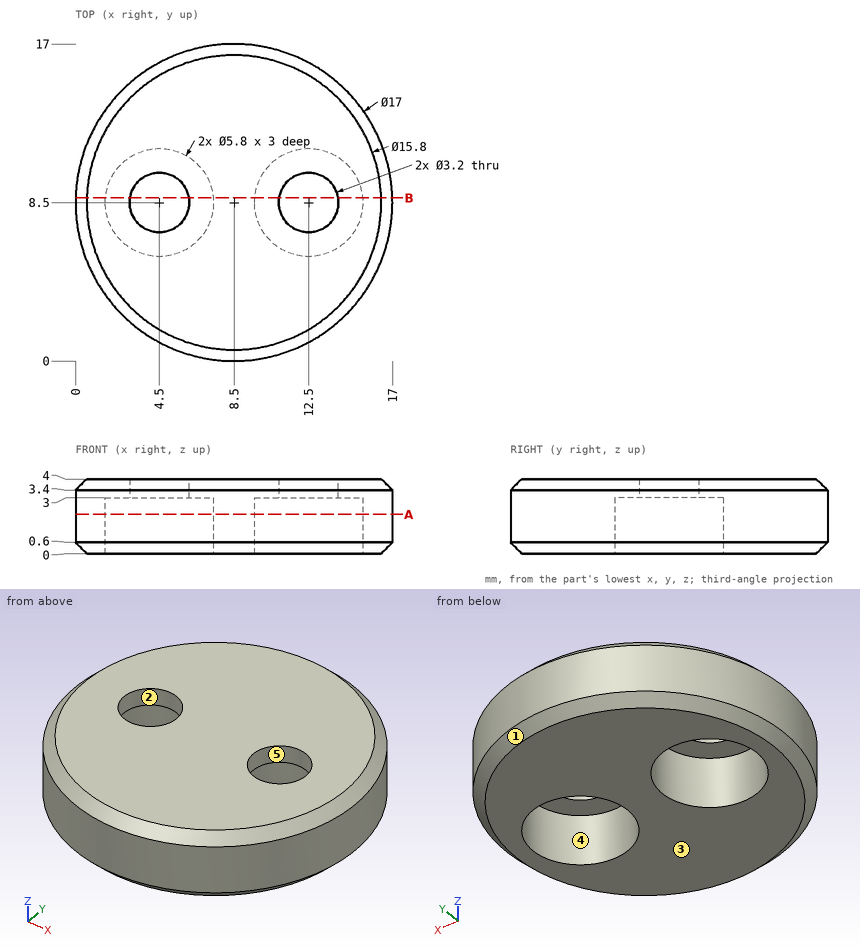
Geometry check sheet. Reference: drawing and pictorial views, mm from the part's lowest x, y, z. A direction names the side the tool comes from. Give positions to 0.01 mm unless a question says otherwise; leave off trailing zeros. Order: outer loops, then holes, each group sorted by start corner. A loop starts at its lowest first (then second) coordinate and runs counter-clockwise, first axis right, second up. Notation, with made-up numbers: M -11.5,-32 L 18.5,-32 A16 ccw 18.5,-1 Z; hole C 39,81.25 d8. An arc over 180 degrees is marked long. Answer as a JSON object with one key per item and string values. Group by question number.
1) Cross-section at A-A (z = 2.1). Enter the section's corners in (x, y).
2) Depth check by flat-ended pin: pin 1 Ø5 at (x, y) = (12.5, 8.5) entering from -Z; pin 2 Ø2 at (x, z) = (5, 2.5) entering from +Y; pin 3 Ø1.5 at (y, z) = (9.5, 0.5) entering from -X. Enter the tip coordinate at first touch or a pass-through.
3) Scan lines: line 1 along X through (y, z) = (7, 2.2); line 2 along X through (y, z) = (6, 2.1); line 3 along Y through (x, z) = (12.5, 1.75). Record each from-to range of solid material in increasing order. Write a range as [from, to].
4) Cross-section at B-B (y = 8.75). Give the number of separate pieces and of enclosed holes in the cut face, then the cut area to 3 significant figures.
5) Access from +Z, -Z, +X, -X, +Y, -Y to the whole of each face (thin tool, end or side, straight path). Record for the marked faces 4 and 5.
6) Mould release check, pull along X, two halves, no side actions. Record for the marked faces 1, 2 and 3: released by +X, released by -X, zero draft, split by the parting line, or undercut.
Result sheet:
{
 "1": {"outline": "C 8.5,8.5 d17; hole C 4.5,8.5 d5.8; hole C 12.5,8.5 d5.8"},
 "2": {"pin 1": "stops at z = 3", "pin 2": "stops at y = 16.62", "pin 3": "stops at x = 0"},
 "3": {"line 1": "x = [0.13, 2.02], [6.98, 10.02], [14.98, 16.87]", "line 2": "x = [0.38, 3.03], [5.97, 11.03], [13.97, 16.62]", "line 3": "y = [1, 5.6], [11.4, 16]"},
 "4": {"separate pieces": "3", "enclosed holes": "0", "area": "26.3 mm2"},
 "5": {"face 4": "-Z", "face 5": "+Z, -Z"},
 "6": {"face 1": "split by the parting line", "face 2": "undercut", "face 3": "zero draft"}
}
